from build123d import *

# Parameters (mm, degrees)
F0_W      = 200
F0_H      = 200
F1_DEPTH  = 15
F2_R      = 20
F3_DEPTH  = 25
F4_DEPTH  = 25
F5_DEPTH  = 26
F6_DEPTH  = 30
F7_DEPTH  = 29
F9_DEPTH  = 25
F11_D     = 9
F12_D     = 7
F14_D     = 5
F14_DEPTH = 20
F14_TIP   = 1.5021515476
F15_DEPTH = 4
F16_DEPTH = 55
F18_DEPTH = 25
F20_D     = 4.2
F20_DEPTH = 15
F20_TIP   = 1.2618073


with BuildPart() as f1:
    # F0 (on Front) → F1 (new body)
    with BuildSketch(Plane.XZ):
        with Locations((100, 100)):
            Rectangle(F0_W, F0_H)
    extrude(amount=F1_DEPTH)

    # F2 (on face) → F3 (cut)
    with BuildSketch(Plane.XZ.offset(15)):
        with Locations((98, 90)):
            Circle(F2_R)
    extrude(amount=-F3_DEPTH, mode=Mode.SUBTRACT)

    # F4 (cut): a face of the model
    f4_faces = [f1.faces().sort_by_distance(p)[0] for p in [
        (100, -7.5, 0),
    ]]
    extrude(f4_faces, amount=-F4_DEPTH, mode=Mode.SUBTRACT)

    # F5 (cut): a face of the model
    f5_faces = [f1.faces().sort_by_distance(p)[0] for p in [
        (100, -7.5, 25),
    ]]
    extrude(f5_faces, amount=-F5_DEPTH, mode=Mode.SUBTRACT)

    # F6 (cut): a face of the model
    f6_faces = [f1.faces().sort_by_distance(p)[0] for p in [
        (0, -7.5, 125.5),
    ]]
    extrude(f6_faces, amount=-F6_DEPTH, mode=Mode.SUBTRACT)

    # F7 (cut): a face of the model
    f7_faces = [f1.faces().sort_by_distance(p)[0] for p in [
        (30, -7.5, 125.5),
    ]]
    extrude(f7_faces, amount=-F7_DEPTH, mode=Mode.SUBTRACT)

    # F8 (on face) → F9 (cut)
    with BuildSketch(Plane.XZ.offset(15)):
        Polygon((200, 51), (200, 61), (190, 51), align=None)
    extrude(amount=-F9_DEPTH, mode=Mode.SUBTRACT)

    # F11 (through all)
    with Locations(Plane.XZ.offset(15)):
        with Locations((180, 100), (180, 140), (180, 180), (140, 180), (140, 140), (140, 100)):
            Hole(F11_D / 2)

    # F12 (through all)
    with Locations(Plane.XZ.offset(15)):
        with Locations((121.5, 66.5), (121.5, 113.5), (74.5, 66.5), (74.5, 113.5)):
            Hole(F12_D / 2)

    # F14
    with Locations(Plane(origin=(0, 0, 51), x_dir=(1, 0, 0), z_dir=(0, 0, -1))):
        with Locations((98, 10)):
            Hole(F14_D / 2, depth=F14_DEPTH)
            with Locations((0, 0, -(F14_DEPTH + F14_TIP / 2))):  # 118° drill point
                Cone(0, F14_D / 2, F14_TIP, mode=Mode.SUBTRACT)

    # F15 (add): a face of the model
    f15_faces = [f1.faces().sort_by_distance(p)[0] for p in [
        (59, -7.5, 125.5),
    ]]
    extrude(f15_faces, amount=F15_DEPTH)

    # F16 (add): a face of the model
    f16_faces = [f1.faces().sort_by_distance(p)[0] for p in [
        (55, -7.5, 125.5),
    ]]
    extrude(f16_faces, amount=F16_DEPTH)

    # F17 (on face) → F18 (cut)
    with BuildSketch(Plane.XZ.offset(15)):
        Polygon((0, 111), (0, 51), (40, 51), align=None)
    extrude(amount=-F18_DEPTH, mode=Mode.SUBTRACT)

    # F20
    with Locations(Plane.XY.offset(200)):
        with Locations((28, -7.5), (61, -7.5), (94, -7.5), (127, -7.5), (160, -7.5)):
            Hole(F20_D / 2, depth=F20_DEPTH)
            with Locations((0, 0, -(F20_DEPTH + F20_TIP / 2))):  # 118° drill point
                Cone(0, F20_D / 2, F20_TIP, mode=Mode.SUBTRACT)


solid = f1.part
Geometry: final body of the model. Coordinates: model frame, mm. A direction names the side the tool comes from. Give positions to 0.01 mm unless a question says otherwise; leave off trailing zeros. Write each loop counter-clockwise with the first axis right and the second up, starting at its lowest first coordinate (ties: lowest second). Pieces come first, ordered by that corner, then holes. Notation, with made-up numbers: M 11,89.5 L 68,89.5 A21 cw 68,111.5 Z; hole C 89.5,21.25 d5. An arc over 180 degrees is marked long. Answer in a Markdown table with one row per item. Add a question column.
(1) Ray query, line 1 (Z direction, x = 140, y = -8.5); line 2 (X direction, y = -7.5, z = 195.75); line 3 (Y direction, x = 28, z = 190). Return the intervals inside material, ascending.
(2) Section A-A on x = 121.5. Return loops of the section in (y, z).
(3) Section B-B on x = 180. Return loops of the section in (y, z).
(4) Section C-C on z = 74.5. Return loops of the section in (x, y).
(5) Reachability of faces 1 (the cylindrical face through (100, -8.5, 60.7)), 2 (the cylindrical face through (118.267, -7.395, 65.159)), 3 (the cylindrical face through (96.1, -7.41, 192.4)) from +Z, -Z, +X, -X, +Y, -Y: full face, straight path, thin tool, end or side. Return the list, or none.
(6) Section D-D on y = -2.75. State how many separate pieces and enclosed holes the cut face has, and give its area (3 significant figures).
(7) First-contact query: pin 1 (4 mm diameter, centred on x = 98, y = -10, fed in from -Z); pin 2 (4 mm diameter, centred on x = 61, y = -7.5, fed in from +Z). Flat tips, straight axial feed; report the tip coordinate or a pass-through.
(8) Mould query, pull axis X, two halves, no side actions, for faces 4 (the cylindrical face through (71.267, -7.395, 112.159)), 5 (the flat face through (101, -15, 124)), 6 (the cylindrical face through (71.267, -7.395, 65.159)), 7 (the flat face through (195, -8, 56)). Classes: +X half, -X half, draft (parallel to the pull), parting line (faces both ways), or undercut.
Result set:
| question | item | result |
|---|---|---|
| 1 | line 1 | z = 51 to 95.5, 104.5 to 135.5, 144.5 to 175.5, 184.5 to 200 |
| 1 | line 2 | x = 0 to 25.9, 30.1 to 58.9, 63.1 to 91.9, 96.1 to 124.9, 129.1 to 157.9, 162.1 to 200 |
| 1 | line 3 | y = -15 to -9.6, -5.4 to 0 |
| 2 | outline | M -15,51 L 0,51 L 0,63 L -15,63 Z; M -15,70 L 0,70 L 0,110 L -15,110 Z; M -15,117 L 0,117 L 0,200 L -15,200 Z |
| 3 | outline | M -15,51 L 0,51 L 0,95.5 L -15,95.5 Z; M -15,104.5 L 0,104.5 L 0,135.5 L -15,135.5 Z; M -15,144.5 L 0,144.5 L 0,175.5 L -15,175.5 Z; M -15,184.5 L 0,184.5 L 0,200 L -15,200 Z |
| 4 | outline | M 24.33,-15 L 85.36,-15 L 85.36,0 L 24.33,0 Z; M 110.64,-15 L 200,-15 L 200,0 L 110.64,0 Z |
| 5 | face 1 | -Z |
| 5 | face 2 | +Y, -Y |
| 5 | face 3 | +Z |
| 6 | separate pieces | 1 |
| 6 | enclosed holes | 11 |
| 6 | area | 26,800 mm^2 |
| 7 | pin 1 | stops at z = 109.9 |
| 7 | pin 2 | stops at z = 184.94 |
| 8 | face 4 | undercut |
| 8 | face 5 | draft |
| 8 | face 6 | undercut |
| 8 | face 7 | +X half |
